from build123d import *

# Parameters (mm, degrees)
SKETCH1_R           = 1.5
SKETCH1_R_2         = 11.5
BOSS_EXTRUDE1_DEPTH = 3
BOSS_EXTRUDE2_DEPTH = 51
BOSS_EXTRUDE3_DEPTH = 51
SKETCH11_W          = 1
SKETCH11_H          = 51
BOSS_EXTRUDE4_DEPTH = 5
BOSS_EXTRUDE6_DEPTH = 10
CHAMFER1_SIZE       = 4
BOSS_EXTRUDE7_DEPTH = 29
SKETCH16_W          = 2.75
SKETCH16_H          = 10
BOSS_EXTRUDE8_DEPTH = 4
CHAMFER2_SIZE       = 1
CHAMFER3_SIZE       = 1


with BuildPart() as part:
    # Sketch1 → Boss-Extrude1 (new body)
    with BuildSketch(Plane(origin=(0, 0, 0), x_dir=(1, 0, 0), z_dir=(0, 1, 0))):
        Polygon((-21.15, 17.15), (-17.15, 21.15), (17.15, 21.15), (21.15, 17.15), (21.15, -17.15), (17.15, -21.15), (-17.15, -21.15), (-21.15, -17.15), align=None)
        with Locations(Location((-15.5, 15.5, 0), (0, 0, 270))):
            Circle(SKETCH1_R, mode=Mode.SUBTRACT)
        with Locations(Location((15.5, 15.5, 0), (0, 0, 270))):
            Circle(SKETCH1_R, mode=Mode.SUBTRACT)
        with Locations(Location((15.5, -15.5, 0), (0, 0, 270))):
            Circle(SKETCH1_R, mode=Mode.SUBTRACT)
        with Locations(Location((-15.5, -15.5, 0), (0, 0, 270))):
            Circle(SKETCH1_R, mode=Mode.SUBTRACT)
        with Locations(Location((0, 0, 0), (0, 0, 270))):
            Circle(SKETCH1_R_2, mode=Mode.SUBTRACT)
    extrude(amount=BOSS_EXTRUDE1_DEPTH)

    # Sketch5 → Boss-Extrude2 (add)
    with BuildSketch(Plane(origin=(0, 0, 0), x_dir=(1, 0, 0), z_dir=(0, 1, 0))):
        Polygon((21.15, -17.15), (23.65, -14.65), (23.65, -18.185533906), (18.185533906, -23.65), (-18.185533906, -23.65), (-23.65, -18.185533906), (-23.65, 14.65), (-23.65, 18.185533906), (-18.185533906, 23.65), (18.185533906, 23.65), (23.65, 18.185533906), (23.65, 14.65), (21.15, 17.15), (17.15, 21.15), (-17.15, 21.15), (-21.15, 17.15), (-21.15, -17.15), (-17.15, -21.15), (17.15, -21.15), align=None)
    extrude(amount=BOSS_EXTRUDE2_DEPTH)

    # Sketch9 → Boss-Extrude3 (add)
    with BuildSketch(Plane(origin=(0, 0, 0), x_dir=(1, 0, 0), z_dir=(0, 1, 0))):
        Polygon((-18.185533906, -23.65), (-21, -28.524798271), (21, -28.524798271), (18.185533906, -23.65), align=None)
    extrude(amount=BOSS_EXTRUDE3_DEPTH)

    # Sketch11 → Boss-Extrude4 (add, symmetric)
    with BuildSketch(Plane(origin=(0, 0, 0), x_dir=(0, 0, -1), z_dir=(1, 0, 0))):
        with Locations((24.15, 25.5)):
            Rectangle(SKETCH11_W, SKETCH11_H)
    extrude(amount=BOSS_EXTRUDE4_DEPTH, both=True)

    # Sketch13 → Boss-Extrude6 (add)
    with BuildSketch(Plane(origin=(5, 0, 0), x_dir=(0, 0, -1), z_dir=(1, 0, 0))):
        Polygon((24.65, 80), (34.65, 80), (36.9, 79.181067), (36.9, 78.3382111), (34.65, 77.5192781), (34.65, 76.8584073), (36.9, 76.0394743), (36.9, 75.1966185), (34.65, 74.3776854), (34.65, 73.7168147), (36.9, 72.8978817), (36.9, 72.0550258), (34.65, 71.2360928), (34.65, 70.575222), (36.9, 69.756289), (36.9, 68.9134332), (34.65, 68.0945001), (34.65, 67.4336294), (36.9, 66.6146964), (36.9, 65.7718405), (34.65, 64.9529075), (34.65, 64.2920367), (36.9, 63.4731037), (36.9, 62.6302478), (34.65, 61.8113148), (34.65, 61.1504441), (36.9, 60.3315111), (36.9, 59.4886552), (34.65, 58.6697222), (34.65, 58.0088514), (36.9, 57.1899184), (36.9, 56.3470625), (34.65, 55.5281295), (34.65, 54.8672588), (36.9, 54.0483257), (36.9, 53.2054699), (34.65, 52.3865369), (34.65, 51.7256661), (36.9, 50.9067331), (36.9, 50.0638772), (34.65, 49.2449442), (34.65, 48.5840735), (36.9, 47.7651404), (36.9, 46.9222846), (34.65, 46.1033516), (34.65, 45.4424808), (36.9, 44.6235478), (36.9, 43.7806919), (34.65, 42.9617589), (34.65, 42.3008882), (36.9, 41.4819551), (36.9, 40.6390993), (34.65, 39.8201662), (34.65, 39.1592955), (36.9, 38.3403625), (36.9, 37.4975066), (34.65, 36.6785736), (34.65, 36.0177028), (36.9, 35.1987698), (36.9, 34.355914), (34.65, 33.5369809), (34.65, 32.8761102), (36.9, 32.0571772), (36.9, 31.2143213), (34.65, 30.3953883), (34.65, 29.7345175), (36.9, 28.9155845), (36.9, 28.0727287), (34.65, 27.2537956), (34.65, 26.5929249), (36.9, 25.7739919), (36.9, 24.931136), (34.65, 24.112203), (34.65, 23.4513322), (36.9, 22.6323992), (36.9, 21.7895434), (34.65, 20.9706103), (34.65, 20.3097396), (36.9, 19.4908066), (36.9, 18.6479507), (34.65, 17.8290177), (34.65, 17.1681469), (36.9, 16.3492139), (36.9, 15.506358), (34.65, 14.687425), (34.65, 14.0265543), (36.9, 13.2076212), (36.9, 12.3647654), (34.65, 11.5458324), (34.65, 10.8849616), (36.9, 10.0660286), (36.9, 9.2231727), (34.65, 8.4042397), (34.65, 7.743369), (36.9, 6.9244359), (36.9, 6.0815801), (34.65, 5.2626471), (34.65, 4.6017763), (36.9, 3.7828433), (36.9, 2.9399874), (34.65, 2.1210544), (34.65, 1.4601837), (36.9, 0.6412506), (36.9, 0), (24.65, 0), align=None)
    extrude(amount=-BOSS_EXTRUDE6_DEPTH)

    # Chamfer1
    chamfer1_edges = [part.edges().sort_by_distance(p)[0] for p in [
        (5, 25.5, -23.65),
    ]]
    chamfer(chamfer1_edges, length=CHAMFER1_SIZE)
    chamfer1_2_edges = [part.edges().sort_by_distance(p)[0] for p in [
        (-5, 25.5, -23.65),
    ]]
    chamfer(chamfer1_2_edges, length=CHAMFER1_SIZE)

    # Sketch15 → Boss-Extrude7 (add)
    with BuildSketch(Plane(origin=(0, 51, 0), x_dir=(1, 0, 0), z_dir=(0, 1, 0))):
        Polygon((-8, 24.65), (-11.5, 21.15), (11.5, 21.15), (8, 24.65), align=None)
    extrude(amount=BOSS_EXTRUDE7_DEPTH)

    # Sketch16 → Boss-Extrude8 (add)
    with BuildSketch(Plane(origin=(0, 51, 0), x_dir=(1, 0, 0), z_dir=(0, 1, 0))):
        with Locations((-25.025, 0)):
            Rectangle(SKETCH16_W, SKETCH16_H)
    extrude(amount=-BOSS_EXTRUDE8_DEPTH)

    # Chamfer2
    chamfer2_edges = [part.edges().sort_by_distance(p)[0] for p in [
        (-23.65, 47, 0),
    ]]
    chamfer(chamfer2_edges, length=CHAMFER2_SIZE)

    # Chamfer3
    chamfer3_edges = [part.edges().sort_by_distance(p)[0] for p in [
        (-23.65, 48.5, -5),
        (-23.65, 48.5, 5),
    ]]
    chamfer(chamfer3_edges, length=CHAMFER3_SIZE)


solid = part.part
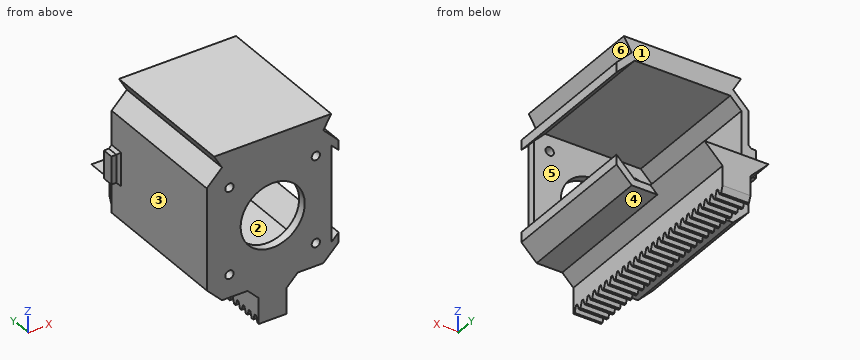
Can you work these out from the model? Positions are in its coordinate system, mm. Face numbers are marked on the shaded views. A direction names the side the tool comes from. Coordinates: 2 decimals unless noted, no trailing zeros. Loops run counter-clockwise (first coordinate to the right, second up) from the corner with the lowest first, then second, coordinate; pieces in that order, holes last. Notation, with made-up numbers: M 70,56.25 L 79,56.25 A31 ccw 79,85.25 Z; hole C 18,-32 d11. An arc over 180 degrees is marked long. Answer as CSV lines item,"result". Start each with the question number.
1. For pin 1 Ø4.5 at (x, y) = (-12, 34.5) entering from -Z; pin 2 Ø2.5 at (x, z) = (16.5, -18) entering from +Y; pin 3 Ø3 at (y, z) = (68.5, -23.5) entering from +X, each with a flat end and sliding along its axis, tell me the tip position at first contact or that it passes through.
2. Suppose I cut it at A-A, the plane z = 0. List the corners of the cut face in (x, y) for me, plus the area to 3 significant figures.
3. If I drill on probe 1 along X at (y, z) = (2, 15.5); probe 2 along Z at (x, y) = (2.5, 19); probe 3 along Z at (x, y) = (-12, 48), over which ranges is the centre line in solid material (lowest first)? Write a range as [from, to].
4. Thinking about a two-plate mould opening in X: for the marked faces 1, 2 and 3, which applies, +X half, -X half, draft (parallel to the pull), parting line (faces both ways), or undercut?
5. For the marked faces 4, 5 and 6, which set-ups out of +Z, -Z, +X, -X, +Y, -Y let a thin tool reach every point of the face, with its end or its side?
6. Suppose I cut it at B-B, the plane x = -15.5. List the corners of the cut face in (y, z) for me.
Output:
1,pin 1,"stops at z = -23.65"
1,pin 2,"stops at y = 3"
1,pin 3,"stops at x = 10.65"
2,outline,"M -26.4,47 L -24.65,47 L -23.65,46 L -23.65,0 L -11.5,0 L -11.5,3 L -21.15,3 L -21.15,51 L -26.4,51 Z; M 11.5,0 L 21.15,0 L 21.15,3 L 11.5,3 Z"
2,area,"197 mm^2"
3,probe 1,"x = [-23.65, -17], [-14, 14], [17, 21.15], [22.8, 23.65]"
3,probe 2,"z = [-36.9, -21.15], [21.15, 28.52]"
3,probe 3,"z = [-23.65, -21.15], [21.15, 28.52]"
4,face 1,"draft"
4,face 2,"undercut"
4,face 3,"-X half"
5,face 4,"-Z, +X, +Y, -Y"
5,face 5,"+Y"
5,face 6,"+X, +Y, -Y"
6,outline,"M 0,-23.65 L 51,-23.65 L 51,-21.15 L 3,-21.15 L 3,-17 L 0,-17 Z; M 0,-14 L 3,-14 L 3,14 L 0,14 Z; M 0,17 L 3,17 L 3,21.15 L 51,21.15 L 51,28.52 L 0,28.52 Z"
